Source: CAD feature listing. Evaluate the final solid. Frame: model axes, mm. A direction names the side the tool comes from. Give positions to 0.01 mm unless a question says otherwise; leave off trailing zeros. Order: outer loops, then holes, each group sorted by start corner. A loop starts at its lowest first (then second) coordinate and runs counter-clockwise, first axis right, second up.
from build123d import *

# Parameters (mm, degrees)
SKETCH1_W           = 120
SKETCH1_H           = 55
BOSS_EXTRUDE1_DEPTH = 3
SKETCH2_W           = 20
SKETCH2_H           = 3
BOSS_EXTRUDE2_DEPTH = 3


with BuildPart() as part:
    # Sketch1 → Boss-Extrude1 (new body)
    with BuildSketch(Plane.XY):
        with Locations((60, 27.5)):
            Rectangle(SKETCH1_W, SKETCH1_H)
    extrude(amount=-BOSS_EXTRUDE1_DEPTH)

    # Sketch2 → Boss-Extrude2 (add)
    with BuildSketch(Plane.XY):
        with Locations((30, -1.5)):
            Rectangle(SKETCH2_W, SKETCH2_H)
        with Locations((90, -1.5)):
            Rectangle(SKETCH2_W, SKETCH2_H)
    extrude(amount=-BOSS_EXTRUDE2_DEPTH)


solid = part.part
1) Ray query, L1, parallel to Y at x = 15, z = -0.3. Return the intervals inside material, ascending.
Checks:
L1: y = 0 to 55
2) Section query B-B on x = 102.5. Output: boundary loops of the cut face in (y, z).
Checks:
outline: (0, -3) - (55, -3) - (55, 0) - (0, 0) - close
3) First-contact query: pin 1 Ø0.9 at (y, z) = (-1.5, -2) entering from +X; pin 2 Ø1.5 at (y, z) = (-1, -1.5) entering from -X. Flat tips, straight axial feed; report the tip coordinate or a pass-through.
Checks:
pin 1: stops at x = 100
pin 2: stops at x = 20
4) Section query A-A on z = -1.3. Output: boundary loops of the cut face in (x, y), and give its area (3 significant figures).
Checks:
outline: (0, 0) - (20, 0) - (20, -3) - (40, -3) - (40, 0) - (80, 0) - (80, -3) - (100, -3) - (100, 0) - (120, 0) - (120, 55) - (0, 55) - close
area: 6,720 mm2
5) Reachability of faces 1 (the face through (59, 55, -1)), 2 (the face through (20, -2, -1)), 3 (the face through (60, 0, -1)), 4 (the face through (90, -3, -1)), 5 (the face through (110, 0, -1)) from +Z, -Z, +X, -X, +Y, -Y: full face, straight path, thin tool, end or side. Return the list, or none.
Checks:
face 1: +Z, -Z, +X, -X, +Y
face 2: +Z, -Z, -X, -Y
face 3: +Z, -Z, -Y
face 4: +Z, -Z, +X, -X, -Y
face 5: +Z, -Z, +X, -Y
